Design review of the part built by this model. Coordinates are the model's own, in mm. Face numbers are marked on the shaded views. A direction names the side the tool comes from. Give positions to 0.01 mm unless a question says otherwise; leave off trailing zeros. Loops run counter-clockwise (first coordinate to the right, second up) from the corner with the lowest first, then second, coordinate; pieces in that order, holes last. Notation, with made-up numbers: (-22.75, 8) - (32.25, 8) arc R26 cw to (32.25, 24) - close; hole circle Ø2 at (-14, 5.5). An arc over 180 degrees is marked (long way). Write each question's results on one line, items separated by ' | '.
```python
from build123d import *

# Parameters (mm, degrees)
BOSS_EXTRUDE1_DEPTH     = 13
SKETCH3_R               = 1
CUT_EXTRUDE1_DEPTH      = 1
CUT_EXTRUDE1_DEPTH_BACK = 16
SKETCH3_4_R             = 1
CUT_EXTRUDE2_DEPTH      = 1
CUT_EXTRUDE2_DEPTH_BACK = 16


with BuildPart() as part:
    # Sketch2 → Boss-Extrude1 (new body)
    with BuildSketch(Plane.XY):
        with BuildLine():
            ThreePointArc((-24, -15), (-24.707106781, -14.707106781), (-25, -14))
            Line((-25, -14), (-25, -1))
            ThreePointArc((-25, -1), (-24.707106781, -0.292893219), (-24, 0))
            Line((-24, 0), (0, 0))
            Line((0, 0), (0, -1))
            Line((0, -1), (-24, -1))
            Line((-24, -1), (-24, -14))
            Line((-24, -14), (0, -14))
            Line((0, -14), (0, -15))
            Line((0, -15), (-24, -15))
        make_face()
    extrude(amount=BOSS_EXTRUDE1_DEPTH)

    # Sketch3 → Cut-Extrude1 (cut, two sides)
    with BuildSketch(Plane(origin=(0, 0, 0), x_dir=(1, 0, 0), z_dir=(0, 1, 0))) as cut_extrude1_sk:
        with Locations((-10, -2.5)):
            Circle(SKETCH3_R)
    extrude(amount=CUT_EXTRUDE1_DEPTH, mode=Mode.SUBTRACT)
    extrude(cut_extrude1_sk.sketch, amount=-CUT_EXTRUDE1_DEPTH_BACK, mode=Mode.SUBTRACT)

    # Sketch3<4> → Cut-Extrude2 (cut, two sides)
    with BuildSketch(Plane(origin=(0, 0, 0), x_dir=(1, 0, 0), z_dir=(0, 1, 0))) as cut_extrude2_sk:
        with Locations((-10, -2.5)):
            Circle(SKETCH3_4_R)
        with Locations((-20, -10.5)):
            Circle(SKETCH3_4_R)
    extrude(amount=CUT_EXTRUDE2_DEPTH, mode=Mode.SUBTRACT)
    extrude(cut_extrude2_sk.sketch, amount=-CUT_EXTRUDE2_DEPTH_BACK, mode=Mode.SUBTRACT)


solid = part.part
```
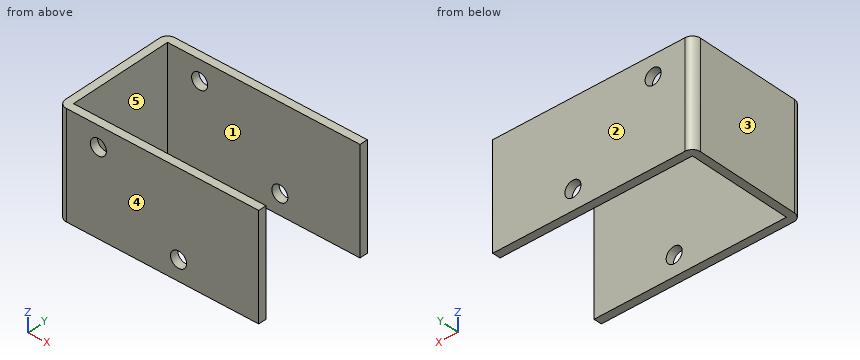
Item 1: Tool access review of the marked faces 1 and 2: name each direction out of +Z, -Z, +X, -X, +Y, -Y from which nothing blocks a thin tool from reaching the whole face with its end or side.
Output values:
face 1: +Z, -Z, +X | face 2: +Z, -Z, +X, -X, +Y
Item 2: Clearance check with flat-ended pins moving along their axes: P1, Ø3, axis at x = -7, z = 10.5, coming from the +Y side; P2, Ø2, axis at y = -3, z = 3.5, coming from the +X side; P3, Ø1.8, axis at x = -20, z = 10.5, coming from the -Y side. State where each tip first meets the part, or that it passes through.
Output values:
P1: stops at y = 0 | P2: stops at x = -24 | P3: passes through
Item 3: We need section D-D on z = 8. Give the boundary of the cut face in (x, y).
Output values:
outline: (-25, -14) arc R1 ccw to (-24, -15) - (0, -15) - (0, -14) - (-24, -14) - (-24, -1) - (0, -1) - (0, 0) - (-24, 0) arc R1 ccw to (-25, -1) - close
Item 4: Draft analysis for pull direction Y (two halves, no side actions). For the marked faces 3, 4 and 5, state which applies: +Y half, -Y half, draft (parallel to the pull), parting line (faces both ways), or undercut.
Output values:
face 3: draft | face 4: -Y half | face 5: undercut
Item 5: We need section B-B on z = 10.5. Give the boundary of the cut face in (x, y).
Output values:
outline: (-25, -14) arc R1 ccw to (-24, -15) - (-21, -15) - (-21, -14) - (-24, -14) - (-24, -1) - (-21, -1) - (-21, 0) - (-24, 0) arc R1 ccw to (-25, -1) - close; (-19, -15) - (0, -15) - (0, -14) - (-19, -14) - close; (-19, -1) - (0, -1) - (0, 0) - (-19, 0) - close
Item 6: Wall thickness on probe 1 along Z at (x, y) = (-20, -14.25); probe 2 along Y at (x, z) = (-22.75, 10.25); probe 3 along Z at (x, y) = (-10, -14.55): over which ranges is each line inside the solid? List them lowest first.
Output values:
probe 1: z = 0 to 9.5, 11.5 to 13 | probe 2: y = -15 to -14, -1 to 0 | probe 3: z = 0 to 1.5, 3.5 to 13
Item 7: We need section A-A on x = -10. Give the boundary of the cut face in (y, z).
Output values:
outline: (-15, 0) - (-14, 0) - (-14, 1.5) - (-15, 1.5) - close; (-15, 3.5) - (-14, 3.5) - (-14, 13) - (-15, 13) - close; (-1, 0) - (0, 0) - (0, 1.5) - (-1, 1.5) - close; (-1, 3.5) - (0, 3.5) - (0, 13) - (-1, 13) - close
Item 8: We need section C-C on x = -14.5. Give the boundary of the cut face in (y, z), then the cut area to 3 significant figures.
Output values:
outline: (-15, 0) - (-14, 0) - (-14, 13) - (-15, 13) - close; (-1, 0) - (0, 0) - (0, 13) - (-1, 13) - close | area: 26.0 mm²
